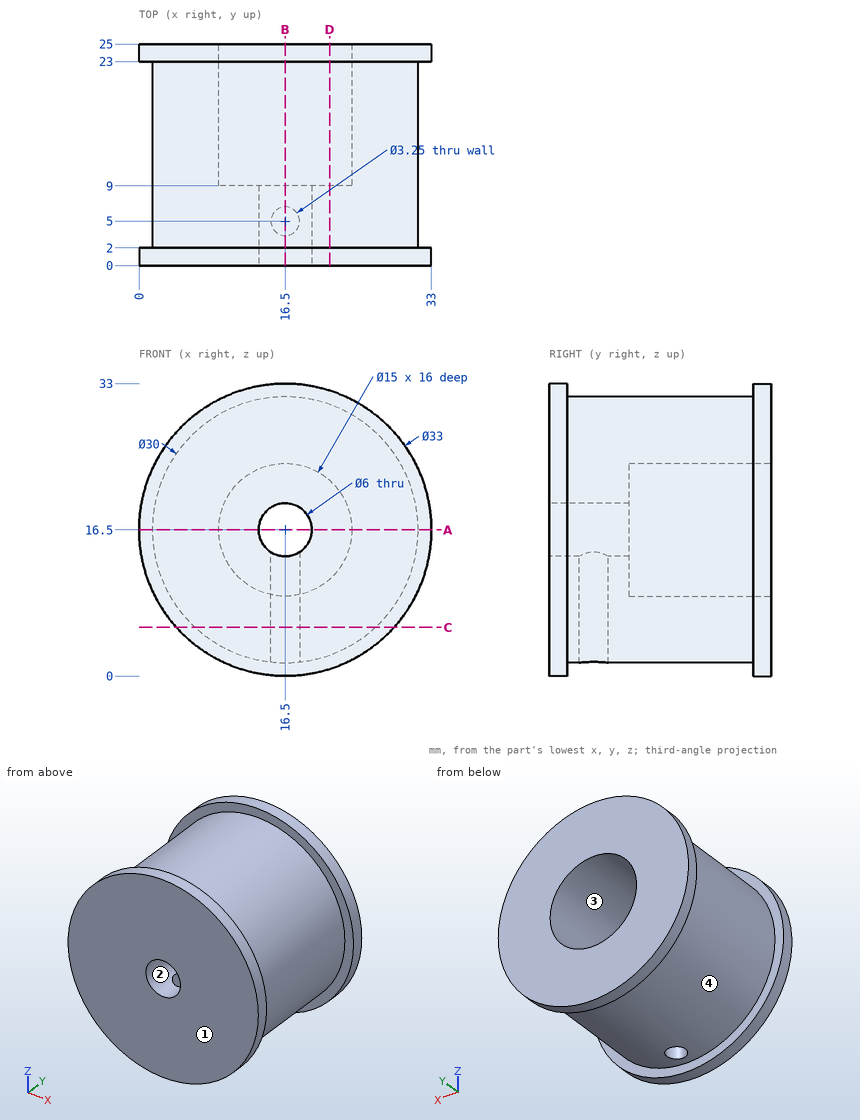
Part print with two shaded views. Sizes in mm from the minimum x, y, z corner. Coordinates: 2 decimals unless noted, no trailing zeros. Write each loop counter-clockwise with the first axis right and the second up, starting at its lowest first coordinate (ties: lowest second). Pieces come first, ordered by that corner, then holes.
(1) Pin check, flat tips, straight feed: pin 1 Ø6 at (y, z) = (7, 27.5) entering from +X; pin 2 Ø1.5 at (y, z) = (21, 5.5) entering from +X; pin 3 Ø5.5 at (x, z) = (16.5, 16.5) entering from +Y; pin 4 Ø1 at (x, y) = (22.5, 11.5) entering from -Z. Stop position of each tip, or through.
(2) Cut at A-A on z = 16.5. List the corners of the cut face in (x, y), and give its area (3 significant figures).
(3) Cut at D-D on x = 21.5. List the corners of the cut face in (y, z), and give its area (3 significant figures).
(4) Drill centre lines: line 1 (Y direction, x = 16.5, z = 4.75) (3 decimals); line 2 (Z direction, x = 16.5, y = 16.5); line 3 (Y direction, x = 16.5, z = 9.25) (3 decimals). Where is each one in solid material? Low to high.
(5) Mould opens along X. For the marked faces 1, 2, 3 and 4 say: pulls with the +X half, pulls with the -X half, needs draft (parallel to the pull), parting line crosses it, or undercut.
(6) Cut at C-C on z = 5.5. List the corners of the cut face in (x, y) (3 decimals).
(7) Cut at B-B on x = 16.5. List the corners of the cut face in (y, z) (3 decimals).
Working result:
1. pin 1: stops at x = 29.19
1. pin 2: stops at x = 27.45
1. pin 3: passes through
1. pin 4: stops at z = 2.54
2. outline: (0, 0) - (13.5, 0) - (13.5, 9) - (9, 9) - (9, 25) - (0, 25) - (0, 23) - (1.5, 23) - (1.5, 2) - (0, 2) - close; (19.5, 0) - (33, 0) - (33, 2) - (31.5, 2) - (31.5, 23) - (33, 23) - (33, 25) - (24, 25) - (24, 9) - (19.5, 9) - close
2. area: 468 mm2
3. outline: (0, 0.78) - (2, 0.78) - (2, 2.36) - (23, 2.36) - (23, 0.78) - (25, 0.78) - (25, 10.91) - (9, 10.91) - (9, 22.09) - (25, 22.09) - (25, 32.22) - (23, 32.22) - (23, 30.64) - (2, 30.64) - (2, 32.22) - (0, 32.22) - close
3. area: 541 mm2
4. line 1: y = 0 to 3.375, 6.625 to 25
4. line 2: z = 1.5 to 9, 24 to 31.5
4. line 3: y = 0 to 3.375, 6.625 to 9
5. face 1: needs draft
5. face 2: undercut
5. face 3: undercut
5. face 4: parting line crosses it
6. outline: (4.202, 0) - (28.798, 0) - (28.798, 2) - (26.698, 2) - (26.698, 23) - (28.798, 23) - (28.798, 25) - (4.202, 25) - (4.202, 23) - (6.302, 23) - (6.302, 2) - (4.202, 2) - close; hole circle Ø3.25 at (16.5, 5)
7. outline: (0, 0) - (2, 0) - (2, 1.5) - (3.375, 1.5) - (3.375, 13.5) - (0, 13.5) - close; (0, 19.5) - (9, 19.5) - (9, 24) - (25, 24) - (25, 33) - (23, 33) - (23, 31.5) - (2, 31.5) - (2, 33) - (0, 33) - close; (6.625, 1.5) - (23, 1.5) - (23, 0) - (25, 0) - (25, 9) - (9, 9) - (9, 13.5) - (6.625, 13.5) - close
